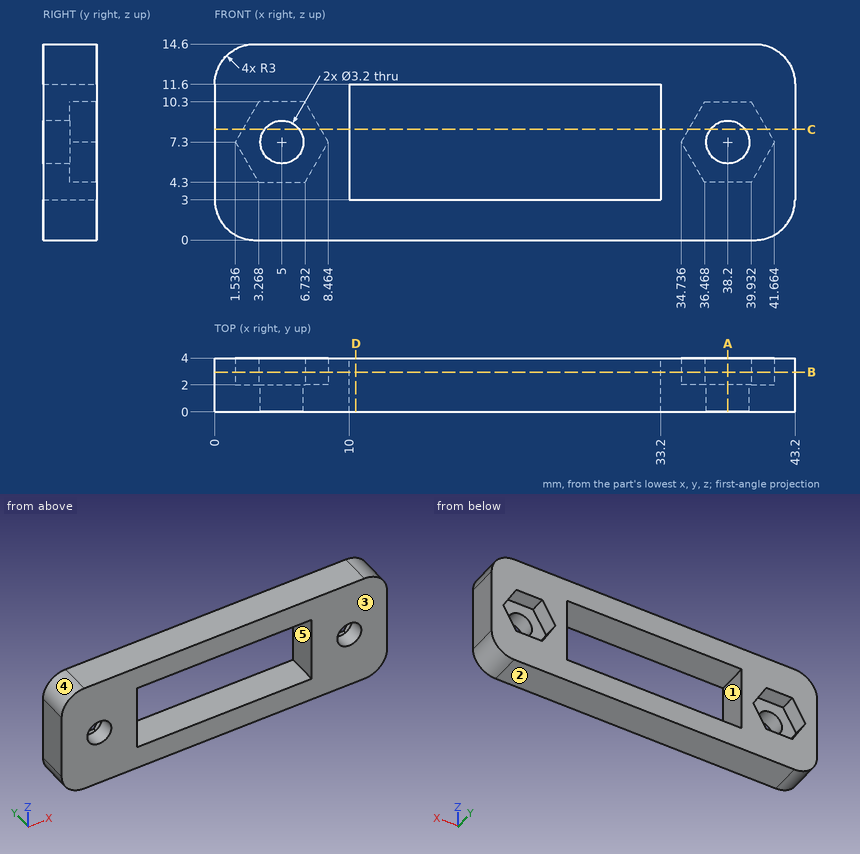
For this review, use the dimensioned drawing (mm, ordinates from the lowest corner) and the shaded views. A direction names the side the tool comes from. Coordinates: 2 decimals unless noted, no trailing zeros. Write each loop counter-clockwise with the first axis right and the second up, starting at its lowest first coordinate (ties: lowest second). Pieces come first, ordered by that corner, then holes. Notation, with made-up numbers: (2, 72.5) - (41, 72.5) arc R24 cw to (41, 88.5) - close; hole circle Ø8 at (40.5, 77). An arc over 180 degrees is marked (long way). Answer as a JSON object with one key per item and string values. Group by question number.
1. Mouldability with a two-part tool opening along Z and no side actions: class the marked faces 3, 4 and 5 as pulls with the +Z half, pulls with the -Z half, needs draft (parallel to the pull), parting line crosses it, or undercut.
2. Add section A-A (x = 38.2). Give the boundary of the cut face in (y, z).
3. Machinability: for the marked faces 1 and 2, which of the approach directions +Z, -Z, +X, -X, +Y, -Y give a long, thin tool a straight path to every point of the face, cutting with its end or side? Answer none if there is none.
4. Clearance check with a flat-ended pin moving along its axis: pin 1 Ø1.8 at (x, z) = (3.5, 8.5) entering from +Y. State where the tip first meets the part, or that it passes through.
5. Add section B-B (y = 2.95). Give the boundary of the cut face in (x, z), plus the area to 3 significant figures.
6. Add section D-D (x = 10.5). Give the boundary of the cut face in (y, z).
7. Add section C-C (z = 8.25). Give the boundary of the cut face in (x, y).
8. To check wall thickness, follow probe 1 along X at (y, z) = (1.2, 7.3); probe 2 along Z at (x, y) = (38.2, 1.05); probe 3 along Z at (x, y) = (5, 3.85). State the ranges of each line that lie inside material, in increasing order.
Findings:
{
 "1": {"face 3": "needs draft", "face 4": "pulls with the +Z half", "face 5": "undercut"},
 "2": {"outline": "(0, 0) - (4, 0) - (4, 4.3) - (2, 4.3) - (2, 5.7) - (0, 5.7) - close; (0, 8.9) - (2, 8.9) - (2, 10.3) - (4, 10.3) - (4, 14.6) - (0, 14.6) - close"},
 "3": {"face 1": "+Y, -Y", "face 2": "-Z, +X, -X, +Y, -Y"},
 "4": {"pin 1": "y = 2"},
 "5": {"outline": "(0, 3) arc R3 ccw to (3, 0) - (40.2, 0) arc R3 ccw to (43.2, 3) - (43.2, 11.6) arc R3 ccw to (40.2, 14.6) - (3, 14.6) arc R3 ccw to (0, 11.6) - close; hole (1.54, 7.3) - (3.27, 4.3) - (6.73, 4.3) - (8.46, 7.3) - (6.73, 10.3) - (3.27, 10.3) - close; hole (10, 3) - (33.2, 3) - (33.2, 11.6) - (10, 11.6) - close; hole (34.74, 7.3) - (36.47, 4.3) - (39.93, 4.3) - (41.66, 7.3) - (39.93, 10.3) - (36.47, 10.3) - close", "area": "361 mm²"},
 "6": {"outline": "(0, 0) - (4, 0) - (4, 3) - (0, 3) - close; (0, 11.6) - (4, 11.6) - (4, 14.6) - (0, 14.6) - close"},
 "7": {"outline": "(0, 0) - (3.71, 0) - (3.71, 2) - (2.08, 2) - (2.08, 4) - (0, 4) - close; (6.29, 0) - (10, 0) - (10, 4) - (7.92, 4) - (7.92, 2) - (6.29, 2) - close; (33.2, 0) - (36.91, 0) - (36.91, 2) - (35.28, 2) - (35.28, 4) - (33.2, 4) - close; (39.49, 0) - (43.2, 0) - (43.2, 4) - (41.12, 4) - (41.12, 2) - (39.49, 2) - close"},
 "8": {"probe 1": "0 to 3.4, 6.6 to 10, 33.2 to 36.6, 39.8 to 43.2", "probe 2": "0 to 5.7, 8.9 to 14.6", "probe 3": "0 to 4.3, 10.3 to 14.6"}
}
